from build123d import *

# Parameters (mm, degrees)
PAD_DEPTH    = 7.5
PAD001_DEPTH = 1.5
FILLET_R     = 1
FILLET001_R  = 0.25
FILLET002_R  = 0.25


with BuildPart() as part:
    # Sketch → Pad (new body)
    with BuildSketch(Plane.XY):
        with BuildLine():
            ThreePointArc((-11.5, 5), (-16.5, 0), (-11.5, -5))
            Line((-11.5, -5), (11.5, -5))
            ThreePointArc((11.5, -5), (16.5, 0), (11.5, 5))
            Line((-11.5, 5), (11.5, 5))
        make_face()
        with BuildLine():
            ThreePointArc((-11.5, 4), (-15.5, 0), (-11.5, -4))
            Line((-11.5, -4), (11.5, -4))
            ThreePointArc((11.5, -4), (15.5, 0), (11.5, 4))
            Line((-11.5, 4), (11.5, 4))
        make_face(mode=Mode.SUBTRACT)
    extrude(amount=PAD_DEPTH)

    # Sketch001 → Pad001 (join)
    with BuildSketch(Plane.XY):
        with BuildLine():
            ThreePointArc((-11.5, 9), (-20.5, 0), (-11.5, -9))
            Line((-11.5, -9), (11.5, -9))
            ThreePointArc((11.5, -9), (20.5, 0), (11.5, 9))
            Line((-11.5, 9), (11.5, 9))
        make_face()
        with BuildLine():
            ThreePointArc((-11.5, 4), (-15.5, 0), (-11.5, -4))
            Line((-11.5, -4), (11.5, -4))
            ThreePointArc((11.5, -4), (15.5, 0), (11.5, 4))
            Line((-11.5, 4), (11.5, 4))
        make_face(mode=Mode.SUBTRACT)
    extrude(amount=PAD001_DEPTH)

    # Fillet
    fillet_edges = [part.edges().sort_by_distance(p)[0] for p in [
        (0, 9, 0),
        (0, 4, 0),
    ]]
    fillet(fillet_edges, radius=FILLET_R)

    # Fillet001
    fillet001_edges = [part.edges().sort_by_distance(p)[0] for p in [
        (0, -5, 7.5),
        (0, -4, 7.5),
    ]]
    fillet(fillet001_edges, radius=FILLET001_R)

    # Fillet002
    fillet002_edges = [part.edges().sort_by_distance(p)[0] for p in [
        (0, 5, 1.5),
    ]]
    fillet(fillet002_edges, radius=FILLET002_R)


solid = part.part
Geometry check sheet. Reference: the model listing, model coordinates, mm. A direction names the side the tool comes from. Round coordinates to 2 decimals unless told otherwise and drop trailing zeros. Write each loop counter-clockwise with the first axis right and the second up, starting at its lowest first coordinate (ties: lowest second). Pieces come first, ordered by that corner, then holes. Notation, with made-up numbers: (87.5, -20.5) -> (131.5, -20.5) arc R29 ccw to (131.5, 16.5) -> close; hole circle Ø6 at (0, 6). An arc over 180 degrees is marked (long way). One line per item, written item: value. Start each with the question number.
(1) Draft check along Y on faces 1 (the cylindrical face through (-20.498, 0.198, 1.246)), 2 (the cylindrical face through (-15.5, 0.1, 4.1)), 3 (the flat face through (0, 5, 4)), 4 (the flat face through (0, 4, 4)). Enter one of: +Y half, -Y half, draft (parallel to the pull), parting line (faces both ways), or undercut.
(2) Cross-section at B-B, the plane x = 8.5. Record the cut outline in (y, z).
(3) Scan lines: line 1 (Y direction, x = -10, z = 4); line 2 (X direction, y = 0, z = 4.75); line 3 (Y direction, x = 14, z = 6.5). Record each from-to range of solid material in increasing order. Write a range as [from, to].
(4) Go/stop test with flat-tipped pins: pin 1 Ø4 at (y, z) = (5.5, 6) entering from +X; pin 2 Ø1.5 at (y, z) = (0, 4) entering from +X; pin 3 Ø3 at (x, z) = (4.5, 3.5) entering from +Y. Record where each tip stops, or that it passes through.
(5) Cross-section at C-C, the plane z = 3.25. Record the cut outline in (x, y), and give its area (3 significant figures).
(6) Access from +Z, -Z, +X, -X, +Y, -Y to the whole of each face (thin tool, end or side, straight path). Record for faces 5 (the cylindrical face through (16.5, -0.1, 4.5)), 6 (the cylindrical face through (-16.5, 0.1, 4.5)), 7 (the flat face through (0, -5, 4)).
(7) Cross-section at A-A, the plane y = 0. Record the cut outline in (x, z).
Answer:
1. face 1: parting line
1. face 2: undercut
1. face 3: +Y half
1. face 4: undercut
2. outline: (-9, 1) arc R1 ccw to (-8, 0) -> (-5, 0) arc R1 ccw to (-4, 1) -> (-4, 7.25) arc R0.25 ccw to (-4.25, 7.5) -> (-4.75, 7.5) arc R0.25 ccw to (-5, 7.25) -> (-5, 1.75) arc R0.25 cw to (-5.25, 1.5) -> (-9, 1.5) -> close; (4, 1) arc R1 ccw to (5, 0) -> (8, 0) arc R1 ccw to (9, 1) -> (9, 1.5) -> (5.25, 1.5) arc R0.25 cw to (5, 1.75) -> (5, 7.25) arc R0.25 ccw to (4.75, 7.5) -> (4.25, 7.5) arc R0.25 ccw to (4, 7.25) -> close
3. line 1: [-5, -4], [4, 5]
3. line 2: [-16.5, -15.5], [15.5, 16.5]
3. line 3: [-4.33, -3.12], [3.12, 4.33]
4. pin 1: x = 15.07
4. pin 2: x = 16.5
4. pin 3: y = 5
5. outline: (-11.5, -5) -> (11.5, -5) arc R5 ccw to (11.5, 5) -> (-11.5, 5) arc R5 ccw to start; hole (-11.5, -4) -> (11.5, -4) arc R4 ccw to (11.5, 4) -> (-11.5, 4) arc R4 ccw to start
5. area: 74.3 mm²
6. face 5: +Z, +X
6. face 6: +Z, -X
6. face 7: +Z, +X, -X, -Y
7. outline: (-20.5, 1) arc R1 ccw to (-19.5, 0) -> (-16.5, 0) arc R1 ccw to (-15.5, 1) -> (-15.5, 7.25) arc R0.25 ccw to (-15.75, 7.5) -> (-16.25, 7.5) arc R0.25 ccw to (-16.5, 7.25) -> (-16.5, 1.75) arc R0.25 cw to (-16.75, 1.5) -> (-20.5, 1.5) -> close; (15.5, 1) arc R1 ccw to (16.5, 0) -> (19.5, 0) arc R1 ccw to (20.5, 1) -> (20.5, 1.5) -> (16.75, 1.5) arc R0.25 cw to (16.5, 1.75) -> (16.5, 7.25) arc R0.25 ccw to (16.25, 7.5) -> (15.75, 7.5) arc R0.25 ccw to (15.5, 7.25) -> close
